```python
from build123d import *

# Parameters (mm, degrees)
SKETCH_W          = 51
SKETCH_H          = 10
SKETCH_R          = 1.65
PAD_DEPTH         = 2
SKETCH001_W       = 39
SKETCH001_H       = 10
PAD001_DEPTH      = 2
POCKET_DEPTH      = 2.001
POCKET_DEPTH_BACK = -2.001
FILLET_R          = 10
FILLET001_R       = 0.5
FILLET002_R       = 3


with BuildPart() as part:
    # Sketch → Pad (new body)
    with BuildSketch(Plane.XY):
        Rectangle(SKETCH_W, SKETCH_H)
        with Locations((-23, 0)):
            Circle(SKETCH_R, mode=Mode.SUBTRACT)
        with Locations((23, 0)):
            Circle(SKETCH_R, mode=Mode.SUBTRACT)
    extrude(amount=-PAD_DEPTH)

    # Sketch001 → Pad001 (join)
    with BuildSketch(Plane.XY):
        Rectangle(SKETCH001_W, SKETCH001_H)
    extrude(amount=PAD001_DEPTH)

    # Sketch002 → Pocket (cut, two sides)
    with BuildSketch(Plane.XY) as pocket_sk:
        Polygon((-10.185143, 3.55), (4.814857, 3.55), (23.608709, 10.390403), (23.793852, 9.340403), (5, 2.5), (-10.185143, 2.5), align=None)
        Polygon((-10.185143, -2.5), (5, -2.5), (23.793852, -9.340403), (23.608709, -10.390403), (4.814857, -3.55), (-10.185143, -3.55), align=None)
    extrude(amount=-POCKET_DEPTH, mode=Mode.SUBTRACT)
    extrude(pocket_sk.sketch, amount=-POCKET_DEPTH_BACK, mode=Mode.SUBTRACT)

    # Fillet
    fillet_edges = [part.edges().sort_by_distance(p)[0] for p in [
        (4.814857, -3.55, 0),
        (5, -2.5, 0),
        (5, 2.5, 0),
        (4.814857, 3.55, 0),
        (11.868694, -5, -1),
        (11.868694, 5, -1),
    ]]
    fillet(fillet_edges, radius=FILLET_R)

    # Fillet001
    fillet001_edges = [part.edges().sort_by_distance(p)[0] for p in [
        (8.798699, -5, -1),
        (8.798699, 5, -1),
        (-10.185143, -3.55, 0),
        (-10.185143, -2.5, 0),
        (-10.185143, 2.5, 0),
        (-10.185143, 3.55, 0),
    ]]
    fillet(fillet001_edges, radius=FILLET001_R)

    # Fillet002
    fillet002_edges = [part.edges().sort_by_distance(p)[0] for p in [
        (-25.5, -5, -1),
        (-25.5, 5, -1),
        (25.5, 5, -1),
        (25.5, -5, -1),
        (19.5, 5, 1),
        (19.5, -5, 1),
        (-19.5, 5, 1),
        (-19.5, -5, 1),
    ]]
    fillet(fillet002_edges, radius=FILLET002_R)


solid = part.part
```
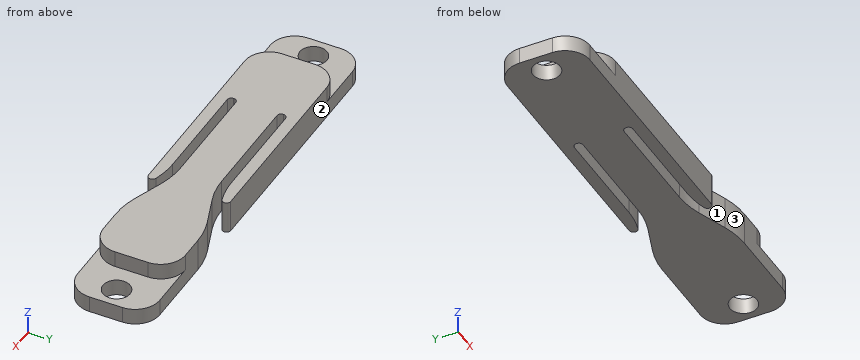
Input: part model. Units: mm. Frame: model coordinates. Face numbers are marked on the shaded views. Round coordinates to 2 decimals unless told otherwise and drop trailing zeros. Loops run counter-clockwise (first coordinate to the right, second up) from the corner with the lowest first, then second, coordinate; pieces in that order, holes last. Notation, with made-up numbers: M 83.25,33 L 115.25,33 A16 cw 115.25,44 Z; hole C 63.5,33 d11. An arc over 180 degrees is marked long. Answer in a Markdown table with one row per item. Add a question column.
1. Ray query, probe 1 along Y at (x, z) = (1, -1.65); probe 2 along X at (y, z) = (-2.25, -0.9); probe 3 along Y at (x, z) = (-23, -0.45). Return the intervals inside material, ascending.
2. Mould query, pull axis X, two halves, no side actions, for the marked faces 1, 2 and 3. Classes: released by +X, released by -X, zero draft, split by the parting line, or undercut.
3. Section B-B (x = -7.5). Output: boundary loops of the cut face in (y, z).
4. Contact query for flat-ended pins moving along their axis: pin 1 (2 mm diameter, centred on x = -23, y = 0, fed in from -Z); pin 2 (1.6 mm diameter, centred on y = -0.5, z = 0.5, fed in from +X); pin 3 (0.6 mm diameter, centred on y = 0.5, z = 1, fed in from -X). Output: stop coordinate, or through.
5. Section A-A (y = 0). Output: boundary loops of the cut face in (x, z), and give its area (3 significant figures).
6. Section D-D (z = -1.45). Give the number of separate pieces and of enclosed holes in the cut face, and give its area (3 significant figures).
7. Section C-C (x = 23). Output: boundary loops of the cut face in (y, z).
Values follow:
| question | item | result |
|---|---|---|
| 1 | probe 1 | -5 to -3.55, -2.5 to 2.5, 3.55 to 5 |
| 1 | probe 2 | -25.49 to 25.49 |
| 1 | probe 3 | -4.96 to -1.65, 1.65 to 4.96 |
| 2 | face 1 | undercut |
| 2 | face 2 | zero draft |
| 2 | face 3 | undercut |
| 3 | outline | M -5,-2 L -3.55,-2 L -3.55,2 L -5,2 Z; M -2.5,-2 L 2.5,-2 L 2.5,2 L -2.5,2 Z; M 3.55,-2 L 5,-2 L 5,2 L 3.55,2 Z |
| 4 | pin 1 | through |
| 4 | pin 2 | x = 25.5 |
| 4 | pin 3 | x = -19.5 |
| 5 | outline | M -25.5,-2 L -24.65,-2 L -24.65,0 L -25.5,0 Z; M -21.35,-2 L 21.35,-2 L 21.35,0 L 19.5,0 L 19.5,2 L -19.5,2 L -19.5,0 L -21.35,0 Z; M 24.65,-2 L 25.5,-2 L 25.5,0 L 24.65,0 Z |
| 5 | area | 167 mm^2 |
| 6 | separate pieces | 1 |
| 6 | enclosed holes | 2 |
| 6 | area | 439 mm^2 |
| 7 | outline | M -4.96,-2 L -1.65,-2 L -1.65,0 L -4.96,0 Z; M 1.65,-2 L 4.96,-2 L 4.96,0 L 1.65,0 Z |
